from build123d import *

# Parameters (mm, degrees)
SKETCH1_W           = 3.175
SKETCH1_H           = 47.625
SKETCH1_H_2         = 3.175
SKETCH1_W_2         = 15.875
BOSS_EXTRUDE1_DEPTH = 184.15
SKETCH2_R           = 2.4892
CUT_EXTRUDE1_DEPTH  = 184.15
CUT_EXTRUDE2_DEPTH  = 165.1


with BuildPart() as part:
    # Sketch1 → Boss-Extrude1 (new body)
    with BuildSketch(Plane.XY):
        with Locations((1.5875, 26.9875)):
            Rectangle(SKETCH1_W, SKETCH1_H)
        with Locations((1.5875, 1.5875)):
            Rectangle(SKETCH1_W, SKETCH1_H_2)
        with Locations((11.1125, 1.5875)):
            Rectangle(SKETCH1_W_2, SKETCH1_H_2)
    extrude(amount=BOSS_EXTRUDE1_DEPTH)

    # Sketch2 → Cut-Extrude1 (cut)
    with BuildSketch(Plane(origin=(0, 3.175, 0), x_dir=(1, 0, 0), z_dir=(0, 1, 0))):
        with Locations(Location((9.525, -6.35, 0), (0, 0, 270))):
            Circle(SKETCH2_R)
        with Locations(Location((9.525, -25.4, 0), (0, 0, 270))):
            Circle(SKETCH2_R)
        with Locations(Location((9.525, -44.45, 0), (0, 0, 270))):
            Circle(SKETCH2_R)
        with Locations(Location((9.525, -63.5, 0), (0, 0, 270))):
            Circle(SKETCH2_R)
        with Locations(Location((9.525, -82.55, 0), (0, 0, 270))):
            Circle(SKETCH2_R)
        with Locations(Location((9.525, -101.6, 0), (0, 0, 270))):
            Circle(SKETCH2_R)
        with Locations(Location((9.525, -120.65, 0), (0, 0, 270))):
            Circle(SKETCH2_R)
        with Locations(Location((9.525, -139.7, 0), (0, 0, 270))):
            Circle(SKETCH2_R)
        with Locations(Location((9.525, -158.75, 0), (0, 0, 270))):
            Circle(SKETCH2_R)
        with Locations(Location((9.525, -177.8, 0), (0, 0, 270))):
            Circle(SKETCH2_R)
    extrude(amount=-CUT_EXTRUDE1_DEPTH, mode=Mode.SUBTRACT)

    # Sketch3 → Cut-Extrude2 (cut)
    with BuildSketch(Plane.ZY):
        with BuildLine():
            Line((76.2, 42.8625), (107.95, 42.8625))
            ThreePointArc((107.95, 42.8625), (112.7125, 38.1), (107.95, 33.3375))
            Line((107.95, 33.3375), (76.2, 33.3375))
            ThreePointArc((76.2, 33.3375), (71.4375, 38.1), (76.2, 42.8625))
        make_face()
    extrude(amount=-CUT_EXTRUDE2_DEPTH, mode=Mode.SUBTRACT)


solid = part.part
Geometry: final body of the model. Coordinates: model frame, mm. A direction names the side the tool comes from. Coordinates: 2 decimals unless noted, no trailing zeros. Write each loop counter-clockwise with the first axis right and the second up, starting at its lowest first coordinate (ties: lowest second). Pieces come first, ordered by that corner, then holes. Notation, with made-up numbers: (19, 15.5) - (42, 15.5) arc R19 cw to (42, 38.5) - close; hole circle Ø11 at (76, 53). An arc over 180 degrees is marked (long way). Return JSON: item names as keys, results as strings.
Item 1: Pin query (flat end, axial travel): pin 1 Ø4.5 at (x, z) = (9.525, 139.7) entering from +Y; pin 2 Ø1 at (y, z) = (16, 153) entering from +X (3 decimals); pin 3 Ø5 at (x, z) = (12, 129.5) entering from +Y (3 decimals). Return the tip coordinate at first contact, or that it passes through.
Completed:
{"pin 1": "passes through", "pin 2": "stops at x = 3.175", "pin 3": "stops at y = 3.175"}
Item 2: Section query A-A (z = 44.45). Output: boundary loops of the cut face in (x, y) (3 decimals).
Completed:
{"outline": "(0, 0) - (7.036, 0) - (7.036, 3.175) - (3.175, 3.175) - (3.175, 50.8) - (0, 50.8) - close; (12.014, 0) - (19.05, 0) - (19.05, 3.175) - (12.014, 3.175) - close"}
Item 3: Line query: L1, parallel to X at y = 2, z = 44.45; L2, parallel to Y at x = 15.75, z = 151.5 (3 decimals). Output: solid intervals per line, ascending.
Completed:
{"L1": "x = 0 to 7.04, 12.01 to 19.05", "L2": "y = 0 to 3.175"}
Item 4: Section query D-D (y = 8.5). Output: boundary loops of the cut face in (x, z) (3 decimals), and give its area (3 significant figures).
Completed:
{"outline": "(0, 0) - (3.175, 0) - (3.175, 184.15) - (0, 184.15) - close", "area": "585 mm2"}
Item 5: Pull-direction query (Y, two-part tool) for faces 3 (the face through (11, 3.175, 91)), 4 (the face through (1.57, 38.2, 112.71)), 5 (the face through (2, 42.862, 92)), 6 (the face through (9.634, 1.61, 61.013)); classes: +Y half, -Y half, draft (parallel to the pull), parting line (faces both ways), or undercut.
Completed:
{"face 3": "+Y half", "face 4": "undercut", "face 5": "undercut", "face 6": "draft"}
Item 6: Section query C-C (z = 82.55). Count the separate pieces of the cut face and the enclosed holes in it, and give its area (3 significant figures).
Completed:
{"separate pieces": "3", "enclosed holes": "0", "area": "166 mm2"}
Item 7: Reachability of faces 1 (the face through (10.273, 1.61, 180.174)), 2 (the face through (1.57, 38, 71.44)) from +Z, -Z, +X, -X, +Y, -Y: full face, straight path, thin tool, end or side. Return the list, or none.
Completed:
{"face 1": "+Y, -Y", "face 2": "+X, -X"}
